```python
from build123d import *

# Parameters (mm, degrees)
SKETCH_W        = 170
SKETCH_H        = 105
PAD_DEPTH       = 1
SKETCH001_W     = 156
SKETCH001_H     = 91
SKETCH001_W_2   = 155
SKETCH001_H_2   = 90
PAD001_DEPTH    = 3
PAD001_FACE16_W = 90
PAD001_FACE16_H = 155
POCKET_DEPTH    = 5


with BuildPart() as part:
    # Sketch → Pad (new body)
    with BuildSketch(Plane.XY):
        Rectangle(SKETCH_W, SKETCH_H)
    extrude(amount=PAD_DEPTH)

    # Sketch001 (on Face6 of Pad) → Pad001 (join)
    with BuildSketch(Plane.XY.offset(1)):
        Rectangle(SKETCH001_W, SKETCH001_H)
        Rectangle(SKETCH001_W_2, SKETCH001_H_2, mode=Mode.SUBTRACT)
    extrude(amount=PAD001_DEPTH)

    # Pad001 Face16 → Pocket (cut)
    with BuildSketch(Plane(origin=(0, 0, 1), x_dir=(0, 1, 0), z_dir=(0, 0, 1))):
        Rectangle(PAD001_FACE16_W, PAD001_FACE16_H)
    extrude(amount=-POCKET_DEPTH, mode=Mode.SUBTRACT)


solid = part.part
```
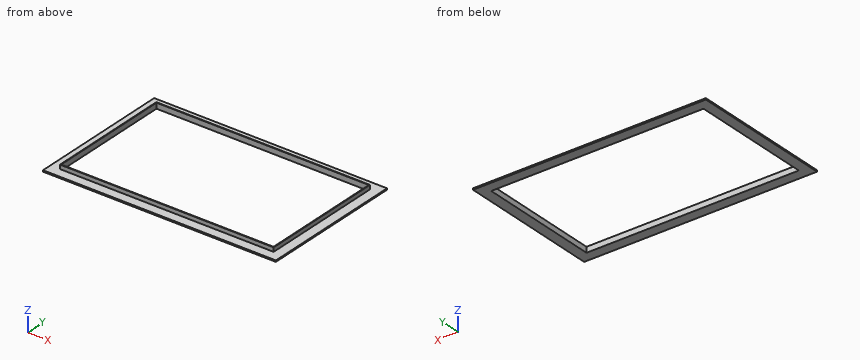
Could you check a few things on this model? Use its own coordinates, in mm. Round coordinates to 2 decimals unless told otherwise and drop trailing zeros. Loops run counter-clockwise (first coordinate to the right, second up) from the corner with the lowest first, then second, coordinate; pieces in that order, holes last.
Q1. For P1, Ø0.9, axis at x = 10, z = 2, coming from the +Y side; P2, Ø1.5, axis at x = 7.5, z = 2, coming from the -Y side; P3, Ø1.2, axis at y = -10, z = 2, coming from the +X side, each with a flat end and sliding along its axis, tell me the tip position at first contact or that it passes through.
Q2. I want a section at A-A (y = 33.5). Write out the boundary of the cut face in (x, z).
Q3. I want a section at B-B (x = -74). Write out the boundary of the cut face in (y, z), and give its area (3 significant figures).
Q4. Please list where these lines run through material, in increasing order: L1, parallel to Y at x = 52, z = 2.15; L2, parallel to X at y = -24.5, z = 1.4; L3, parallel to Y at x = -71.5, z = 0.35.
Q5. I want a section at C-C (z = 2.95). Write out the boundary of the cut face in (x, y).
Answer below:
1. P1: stops at y = 45.5
1. P2: stops at y = -45.5
1. P3: stops at x = 78
2. outline: (-85, 0) - (-77.5, 0) - (-77.5, 4) - (-78, 4) - (-78, 1) - (-85, 1) - close; (77.5, 0) - (85, 0) - (85, 1) - (78, 1) - (78, 4) - (77.5, 4) - close
3. outline: (-52.5, 0) - (-45, 0) - (-45, 4) - (-45.5, 4) - (-45.5, 1) - (-52.5, 1) - close; (45, 0) - (52.5, 0) - (52.5, 1) - (45.5, 1) - (45.5, 4) - (45, 4) - close
3. area: 18.0 mm2
4. L1: y = -45.5 to -45, 45 to 45.5
4. L2: x = -78 to -77.5, 77.5 to 78
4. L3: y = -52.5 to -45, 45 to 52.5
5. outline: (-78, -45.5) - (78, -45.5) - (78, 45.5) - (-78, 45.5) - close; hole (-77.5, -45) - (77.5, -45) - (77.5, 45) - (-77.5, 45) - close
